Part model, mm, in its own coordinate system. Coordinates: 2 decimals unless noted, no trailing zeros. Loops run counter-clockwise (first coordinate to the right, second up) from the corner with the lowest first, then second, coordinate; pieces in that order, holes last. Notation, with made-up numbers: M 47.5,47 L 57.5,47 A18 ccw 57.5,62 Z; hole C -26.75,87.5 d3. An arc over 180 degrees is marked long. Use a Markdown table: item, result. Add a question column.
1) Wall check: probe 1 along Z at (x, y) = (234.95, -3.5); probe 2 along X at (y, z) = (-15.5, 4); probe 3 along Z at (x, y) = (222.25, -15) (3 decimals). Give the ranges that are in metal, low to high. Write a range as from..to.
2) Band-saw the part on A-A (z = 2.75). List the corners of the cut face in (x, y) (3 decimals).
3) Pin check, flat tips, straight feed: pin 1 Ø3.5 at (x, z) = (38.1, 3.175) entering from -Y; pin 2 Ø1.9 at (x, z) = (25.5, 2.5) entering from +Y. Stop position of each tip, or through.
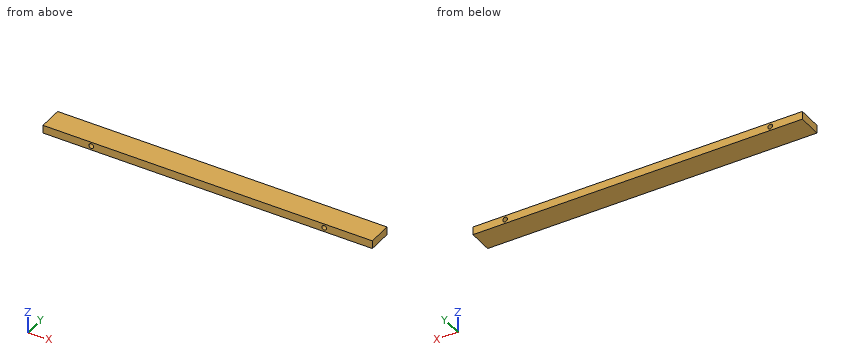
from build123d import *

# Parameters (mm, degrees)
SKETCH1_W           = 260.35
SKETCH1_H           = 19.05
BOSS_EXTRUDE1_DEPTH = 6.35
SKETCH2_R           = 1.88358262
SKETCH2_R_2         = 1.866453282
CUT_EXTRUDE1_DEPTH  = 6.35
SKETCH3_R           = 1.849990648
CUT_EXTRUDE2_DEPTH  = 6.35


with BuildPart() as part:
    # Sketch1 → Boss-Extrude1 (new body)
    with BuildSketch(Plane.XY):
        with Locations((130.175, -9.525)):
            Rectangle(SKETCH1_W, SKETCH1_H)
    extrude(amount=BOSS_EXTRUDE1_DEPTH)

    # Sketch2 → Cut-Extrude1 (cut)
    with BuildSketch(Plane(origin=(0, 0, 0), x_dir=(1, 0, 0), z_dir=(0, 1, 0))):
        with Locations(Location((234.95, -3.175, 0), (0, 0, 270))):
            Circle(SKETCH2_R)
        with Locations(Location((25.4, -3.175, 0), (0, 0, 270))):
            Circle(SKETCH2_R_2)
    extrude(amount=-CUT_EXTRUDE1_DEPTH, mode=Mode.SUBTRACT)

    # Sketch3 → Cut-Extrude2 (cut)
    with BuildSketch(Plane(origin=(0, -19.05, 0), x_dir=(-1, 0, 0), z_dir=(0, -1, 0))):
        with Locations(Location((-222.25, -3.175, 0), (0, 0, 90))):
            Circle(SKETCH3_R)
        with Locations(Location((-38.1, -3.175, 0), (0, 0, 90))):
            Circle(SKETCH3_R)
    extrude(amount=-CUT_EXTRUDE2_DEPTH, mode=Mode.SUBTRACT)


solid = part.part
Entries:
| question | item | result |
|---|---|---|
| 1 | probe 1 | 0..1.29, 5.06..6.35 |
| 1 | probe 2 | 0..36.44, 39.76..220.59, 223.91..260.35 |
| 1 | probe 3 | 0..1.325, 5.025..6.35 |
| 2 | outline | M 0,-19.05 L 36.299,-19.05 L 36.299,-12.7 L 39.901,-12.7 L 39.901,-19.05 L 220.449,-19.05 L 220.449,-12.7 L 224.051,-12.7 L 224.051,-19.05 L 260.35,-19.05 L 260.35,0 L 236.785,0 L 236.785,-6.35 L 233.115,-6.35 L 233.115,0 L 27.217,0 L 27.217,-6.35 L 23.583,-6.35 L 23.583,0 L 0,0 Z |
| 3 | pin 1 | y = -12.7 |
| 3 | pin 2 | y = -6.35 |
